from build123d import *

# Parameters (mm, degrees)
F0_W     = 50.8
F0_H     = 112.817927
F1_DEPTH = 136.387214
F2_R     = 25.4
F3_DEPTH = 25.4
F4_R     = 6.35
F5_R     = 12.7
F6_R     = 12.7


with BuildPart() as f1:
    # F0 (on Top) → F1 (new body)
    with BuildSketch(Plane.XY):
        with Locations((25.4, 56.408963)):
            Rectangle(F0_W, F0_H)
    extrude(amount=F1_DEPTH)

    # F2 (on face) → F3 (join)
    with BuildSketch(Plane.YZ.offset(50.8)):
        with Locations((50.8, 85.587214)):
            Circle(F2_R)
    extrude(amount=F3_DEPTH)

    # F4
    f4_edges = [f1.edges().sort_by_distance(p)[0] for p in [
        (76.2, 25.4, 85.587214),
        (50.8, 25.4, 85.587214),
    ]]
    fillet(f4_edges, radius=F4_R)

    # F5
    f5_edges = [f1.edges().sort_by_distance(p)[0] for p in [
        (25.4, 112.817927, 136.387214),
        (25.4, 112.817927, 0),
        (25.4, 0, 0),
        (25.4, 0, 136.387214),
    ]]
    fillet(f5_edges, radius=F5_R)

    # F6
    f6_edges = [f1.edges().sort_by_distance(p)[0] for p in [
        (50.8, 0, 68.193607),
    ]]
    fillet(f6_edges, radius=F6_R)


solid = f1.part
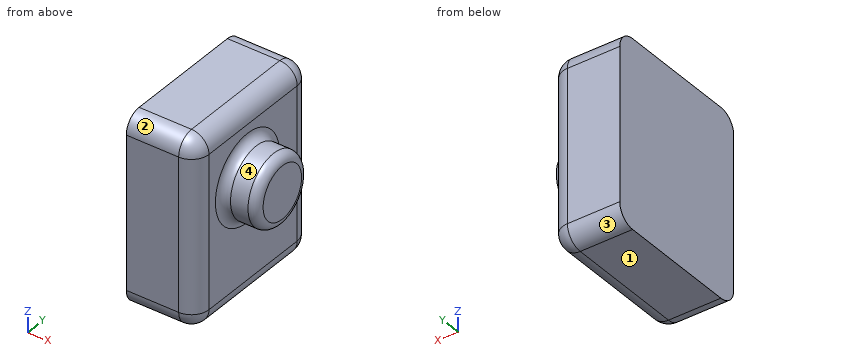
Input: part model. Units: mm. Frame: model coordinates. Face numbers are marked on the shaded views. Give positions to 0.01 mm unless a question says otherwise; leave off trailing zeros. Order: outer loops, then holes, each group sorted by start corner. A loop starts at its lowest first (then second) coordinate and runs counter-clockwise, first axis right, second up. Notation, with made-up numbers: (32.25, 78.5) -> (41.25, 78.5) arc R21 ccw to (41.25, 95.5) -> close; hole circle Ø5 at (-10, 12). An arc over 180 degrees is marked (long way). Use one line per item in the form item = value.
1) Section A-A, the plane y = 50.8. Return loops of the section in (x, z), and give its area (3 significant figures).
Response values:
outline = (0, 0) -> (38.1, 0) arc R12.7 ccw to (50.8, 12.7) -> (50.8, 53.84) arc R6.35 cw to (57.15, 60.19) -> (69.85, 60.19) arc R6.35 ccw to (76.2, 66.54) -> (76.2, 104.64) arc R6.35 ccw to (69.85, 110.99) -> (57.15, 110.99) arc R6.35 cw to (50.8, 117.34) -> (50.8, 123.69) arc R12.7 ccw to (38.1, 136.39) -> (0, 136.39) -> close
area = 8,150 mm^2
2) First-contact query: pin 1 Ø12 at (x, z) = (48.5, 74.5) entering from +Y; pin 2 Ø10 at (x, z) = (45, 44) entering from +Y (3 decimals); pin 3 Ø8 at (y, z) = (51, 38) entering from +X. Flat tips, straight axial feed; report the tip coordinate or a pass-through.
Response values:
pin_1 = 112.03
pin_2 = 112.675
pin_3 = 50.8
3) Line query: probe 1 along X at (y, z) = (24, 12.5); probe 2 along Z at (x, y) = (43, 96); probe 3 along X at (y, z) = (98, 129). Output: solid intervals per line, ascending.
Response values:
probe_1 = 0 to 50.8
probe_2 = 0.98 to 135.4
probe_3 = 0 to 49.64
4) Mould query, pull axis Y, two halves, no side actions, for the marked faces 1, 2, 3 and 4. Classes: pulls with the +Y half, pulls with the -Y half, needs draft (parallel to the pull), parting line crosses it, or undercut.
Response values:
face_1 = needs draft
face_2 = pulls with the -Y half
face_3 = pulls with the +Y half
face_4 = parting line crosses it
5) Section C-C, the plane y = 89.5. Return loops of the section in (x, z), and give its area (3 significant figures).
Response values:
outline = (0, 0) -> (38.1, 0) arc R12.7 ccw to (50.8, 12.7) -> (50.8, 123.69) arc R12.7 ccw to (38.1, 136.39) -> (0, 136.39) -> close
area = 6,860 mm^2
6) Section B-B, the plane x = 46.5. Return loops of the section in (y, z), and give its area (3 significant figures).
Response values:
outline = (3.17, 12.7) arc R9.53 ccw to (12.7, 3.17) -> (100.12, 3.17) arc R9.53 ccw to (109.64, 12.7) -> (109.64, 123.69) arc R9.53 ccw to (100.12, 133.21) -> (12.7, 133.21) arc R9.53 ccw to (3.17, 123.69) -> close
area = 13,800 mm^2
7) Section D-D, the plane x = 67. Return loops of the section in (y, z).
Response values:
outline = circle Ø50.8 at (50.8, 85.59)
